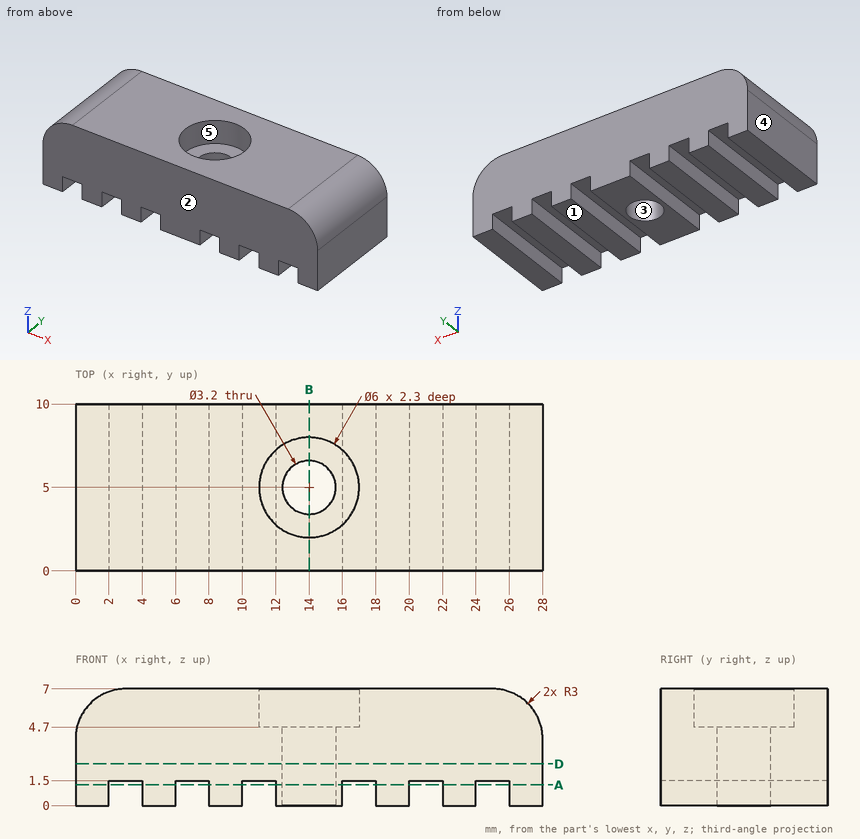
Part print with two shaded views. Sizes in mm from the minimum x, y, z corner. A direction names the side the tool comes from. Coordinates: 2 decimals unless noted, no trailing zeros. Order: outer loops, then holes, each group sorted by start corner. A loop starts at its lowest first (then second) coordinate and runs counter-clockwise, first axis right, second up. Notation, with made-up numbers: (61, 86.25) - (112, 86.25) arc R4 ccw to (112, 91.25) - close; hole circle Ø2 at (-38.75, -34). An arc over 180 degrees is marked (long way). Write item = value, one per line. Start each with the question number.
1) Flat gauge pin, fed straight in: pin 1 Ø1 at (x, y) = (3, 4) entering from -Z. Where does the tip first touch, or does it go through?
2) Two-plate mould, pull along Y, no slides. Class the marked faces 1, 2 and 3: pulls with the +Y half, pulls with the -Y half, needs draft (parallel to the pull), parting line crosses it, or undercut.
3) Saw through at B-B on x = 14. Write the cut outline in (y, z), then the cut area to 3 significant figures.
4) Wall check: line 1 along Y through (x, z) = (14, 5.6); line 2 along Y through (x, z) = (14, 3.6); line 3 along Z through (x, y) = (17.5, 9). Give the ranges that are in metal, low to high. Write a range as from..to.
5) 3-axis set-ups, long thin cutter, end or side, ignore diameter. For the marked faces 4 and 5: which of +Z, -Z, +X, -X, +Y, -Y reach the whole face in a straight line?
6) Saw through at A-A on z = 1.25. Count the separate pieces of the cut face and the enclosed holes in it, then the cut area to 3 significant figures.
7) Saw through at D-D on z = 2.5. Write the cut outline in (x, y).
From the geometry:
q1.pin_1 = 1.5
q2.face_1 = needs draft
q2.face_2 = pulls with the -Y half
q2.face_3 = undercut
q3.outline = (0, 0) - (3.4, 0) - (3.4, 4.7) - (2, 4.7) - (2, 7) - (0, 7) - close; (6.6, 0) - (10, 0) - (10, 7) - (8, 7) - (8, 4.7) - (6.6, 4.7) - close
q3.area = 41.2 mm^2
q4.line_1 = 0..2, 8..10
q4.line_2 = 0..3.4, 6.6..10
q4.line_3 = 1.5..7
q5.face_4 = +Z, -Z, -X, +Y, -Y
q5.face_5 = +Z
q6.separate_pieces = 7
q6.enclosed_holes = 1
q6.area = 152 mm^2
q7.outline = (0, 0) - (28, 0) - (28, 10) - (0, 10) - close; hole circle Ø3.2 at (14, 5)
